Verification items for the finished model (mm, model axes). A direction names the side the tool comes from. Coordinates: 2 decimals unless noted, no trailing zeros. Order: outer loops, then holes, each group sorted by start corner. A loop starts at its lowest first (then second) coordinate and runs counter-clockwise, first axis right, second up. Notation, with made-up numbers: (16, 64) -> (66, 64) arc R23 ccw to (66, 102) -> close; hole circle Ø8 at (35, 56.5). An arc over 180 degrees is marked (long way). Write item = value, one per line. Start each with the question number.
from build123d import *

# Parameters (mm, degrees)
SKETCH2_R          = 0.3937
EXTRUDE1_DEPTH     = 1.1811
CIRPATTERN1_COUNT  = 4
CUT_EXTRUDE1_DEPTH = 2.54


with BuildPart() as part:
    # Sketch2 → Extrude1 (new, symmetric)
    with BuildSketch(Plane.XY):
        with BuildLine():
            Line((-28.40736, 35.5092), (17.044416, 35.5092))
            ThreePointArc((17.044416, 35.5092), (18.048767845, 35.925216155), (18.464784, 36.929568))
            Line((18.464784, 36.929568), (18.464784, 53.2638))
            ThreePointArc((18.464784, 53.2638), (20.336856699, 57.783383301), (24.85644, 59.655456))
            Line((24.85644, 59.655456), (29.117544, 59.655456))
            ThreePointArc((29.117544, 59.655456), (33.637127301, 57.783383301), (35.5092, 53.2638))
            Line((35.5092, 53.2638), (35.5092, 14.20368))
            Line((35.5092, 14.20368), (46.872144, 14.20368))
            Line((46.872144, 14.20368), (46.872144, 71.0184))
            Line((46.872144, 71.0184), (30.30982, 71.0184))
            ThreePointArc((30.30982, 71.0184), (30.220017439, 71.055597439), (30.18282, 71.1454))
            Line((30.18282, 71.1454), (30.18282, 73.1774))
            ThreePointArc((30.18282, 73.1774), (29.88524049, 73.89582049), (29.16682, 74.1934))
            Line((29.16682, 74.1934), (13.44422, 74.1934))
            ThreePointArc((13.44422, 74.1934), (12.72579951, 73.89582049), (12.42822, 73.1774))
            Line((12.42822, 73.1774), (12.42822, 71.1454))
            ThreePointArc((12.42822, 71.1454), (12.391022561, 71.055597439), (12.30122, 71.0184))
            Line((12.30122, 71.0184), (7.10184, 71.0184))
            Line((7.10184, 71.0184), (7.10184, 53.2638))
            ThreePointArc((7.10184, 53.2638), (5.229767301, 48.744216699), (0.710184, 46.872144))
            Line((0.710184, 46.872144), (-28.40736, 46.872144))
            Line((-28.40736, 46.872144), (-28.40736, 35.5092))
        make_face()
        with Locations((19.01952, 72.6694)):
            Circle(SKETCH2_R, mode=Mode.SUBTRACT)
        with Locations((23.59152, 72.6694)):
            Circle(SKETCH2_R, mode=Mode.SUBTRACT)
    extrude1 = extrude(amount=EXTRUDE1_DEPTH, both=True)

    # CirPattern1: Extrude1 ×4 about axis
    cirpattern1_axis = Axis((0, 0, 0), (0, 0, 1))
    for i in range(1, CIRPATTERN1_COUNT):
        add(extrude1.rotate(cirpattern1_axis, i * 360 / CIRPATTERN1_COUNT))

    # Sketch3 → Cut-Extrude1 (cut)
    with BuildSketch(Plane.XY.offset(1.1811)):
        with BuildLine():
            Line((29.117544, 60.099956), (24.85644, 60.099956))
            ThreePointArc((24.85644, 60.099956), (20.022547735, 58.097692265), (18.020284, 53.2638))
            Line((18.020284, 53.2638), (18.020284, 36.929568))
            ThreePointArc((18.020284, 36.929568), (17.73445888, 36.23952512), (17.044416, 35.9537))
            Line((17.044416, 35.9537), (-53.2638, 35.9537))
            ThreePointArc((-53.2638, 35.9537), (-58.097692265, 33.951436265), (-60.099956, 29.117544))
            Line((-60.099956, 29.117544), (-60.099956, 24.85644))
            ThreePointArc((-60.099956, 24.85644), (-58.097692265, 20.022547735), (-53.2638, 18.020284))
            Line((-53.2638, 18.020284), (-36.929568, 18.020284))
            ThreePointArc((-36.929568, 18.020284), (-36.23952512, 17.73445888), (-35.9537, 17.044416))
            Line((-35.9537, 17.044416), (-35.9537, -53.2638))
            ThreePointArc((-35.9537, -53.2638), (-33.951436265, -58.097692265), (-29.117544, -60.099956))
            Line((-29.117544, -60.099956), (-24.85644, -60.099956))
            ThreePointArc((-24.85644, -60.099956), (-20.022547735, -58.097692265), (-18.020284, -53.2638))
            Line((-18.020284, -53.2638), (-18.020284, -36.929568))
            ThreePointArc((-18.020284, -36.929568), (-17.73445888, -36.23952512), (-17.044416, -35.9537))
            Line((-17.044416, -35.9537), (53.2638, -35.9537))
            ThreePointArc((53.2638, -35.9537), (58.097692265, -33.951436265), (60.099956, -29.117544))
            Line((60.099956, -29.117544), (60.099956, -24.85644))
            ThreePointArc((60.099956, -24.85644), (58.097692265, -20.022547735), (53.2638, -18.020284))
            Line((53.2638, -18.020284), (36.929568, -18.020284))
            ThreePointArc((36.929568, -18.020284), (36.23952512, -17.73445888), (35.9537, -17.044416))
            Line((35.9537, -17.044416), (35.9537, 53.2638))
            ThreePointArc((35.9537, 53.2638), (33.951436265, 58.097692265), (29.117544, 60.099956))
        make_face()
    extrude(amount=-CUT_EXTRUDE1_DEPTH, mode=Mode.SUBTRACT)


solid = part.part
Item 1: Section check A-A (y = 9.5). Record the boundary of the cut face in (x, z), then the cut area to 3 significant figures.
Item 2: Mould release check, pull along X, two halves, no side actions. Record for faces 3 (the cylindrical face through (48.794, -5.279, 0.017)), 4 (the cylindrical face through (-48.794, 5.279, 0.017)), 5 (the flat face through (39, 0, 1.181)), 6 (the cylindrical face through (-34.004, -58.044, 0.017)): pulls with the +X half, pulls with the -X half, needs draft (parallel to the pull), parting line crosses it, or undercut.
Item 3: Section check B-B (x = 39). Record the boundary of the cut face in (y, z).
Item 4: Tool access check on faces 1 (the cylindrical face through (34.004, 58.044, 0.017)), 2 (the cylindrical face through (5.279, 48.794, 0.017)). Record the directions out of +Z, -Z, +X, -X, +Y, -Y that give a thin tool (end or side, any length) a straight path to the whole face; none if there is none.
Item 5: Section check D-D (z = 0.5). State how many separate pieces and enclosed holes the cut face has, then the cut area to 3 significant figures.
Item 6: Section check C-C (x = 62.5). Record the boundary of the cut face in (y, z).
Item 7: Gauge pin test, flat ends, axial feed: P1, Ø1, axis at y = -72.5, z = 0, coming from the +X side; P2, Ø1, axis at x = -72, z = -0.5, coming from the +Y side; P3, Ø1.2, axis at x = -60.5, z = -0.5, coming from the -Y side. Record the tip position at first contact, or that the pin passes through.
Item 8: Thickness scan on line 1 (X direction, y = 37.5, z = -0.5); line 2 (Y direction, x = 37.5, z = 0.9). Record the ranges inside material, lowest first.
Filled sheet:
q1.outline = (-71.02, -1.18) -> (-35.95, -1.18) -> (-35.95, 1.18) -> (-71.02, 1.18) -> close; (35.95, -1.18) -> (46.87, -1.18) -> (46.87, 1.18) -> (35.95, 1.18) -> close
q1.area = 109 mm^2
q2.face_3 = pulls with the +X half
q2.face_4 = pulls with the -X half
q2.face_5 = needs draft
q2.face_6 = undercut
q3.outline = (-46.87, -1.18) -> (-35.95, -1.18) -> (-35.95, 1.18) -> (-46.87, 1.18) -> close; (-18.02, -1.18) -> (71.02, -1.18) -> (71.02, 1.18) -> (-18.02, 1.18) -> close
q4.face_1 = +Z, -Z
q4.face_2 = +Z, -Z, -X, +Y
q5.separate_pieces = 1
q5.enclosed_holes = 9
q5.area = 6,060 mm^2
q6.outline = (-46.87, -1.18) -> (-7.1, -1.18) -> (-7.1, 1.18) -> (-46.87, 1.18) -> close
q7.P1 = -12.43
q7.P2 = 30.18
q7.P3 = 7.1
q8.line_1 = -71.02 to 18.02, 35.95 to 46.87
q8.line_2 = -46.87 to -35.95, -18.02 to 71.02
